CAD build for the part. Positions are in the model's coordinates, mm. Face numbers are marked on the shaded views. Round coordinates to 2 decimals unless told otherwise and drop trailing zeros. Order: outer loops, then holes, each group sorted by start corner. A loop starts at its lowest first (then second) coordinate and runs counter-clockwise, first axis right, second up. Notation, with made-up numbers: M -8.75,69.25 L 20.25,69.25 A28 cw 20.25,105.25 Z; hole C 44.25,31 d6. An arc over 180 degrees is marked long. Answer as a JSON object with one key per item and string values.
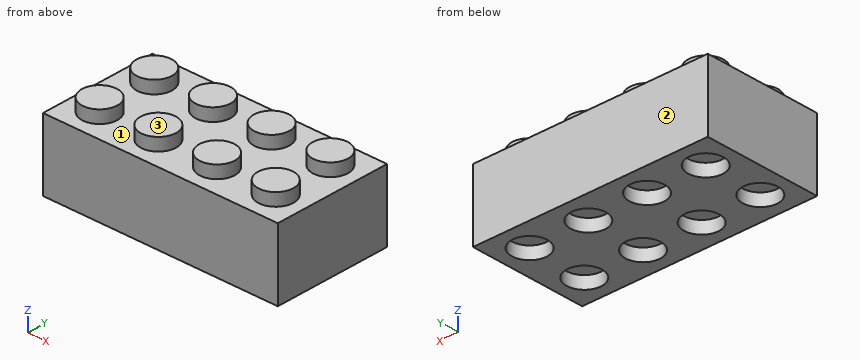
```python
from build123d import *

# Parameters (mm, degrees)
F1_DEPTH = 8
F3_W     = 8
F3_H     = 8
F3_R     = 2.4
F4_DEPTH = 1.7
F5_R     = 2.4
F6_DEPTH = 1.7


with BuildPart() as f1:
    # F0 (on Front) → F1 (new body)
    with BuildSketch(Plane.XZ):
        Polygon((-2.4, 9.6), (-4, 9.6), (-4, 0), (4, 0), (4, 9.6), (2.4, 9.6), (2.4, 11.3), (-2.4, 11.3), align=None)
    extrude(amount=F1_DEPTH)

    # F3 (on plane+point) → F4 (cut, through all)
    with BuildSketch(Plane.XY.offset(11.3)):
        with Locations((0, -4)):
            Rectangle(F3_W, F3_H)
        with Locations((0, -4)):
            Circle(F3_R, mode=Mode.SUBTRACT)
    extrude(amount=-F4_DEPTH, mode=Mode.SUBTRACT)

    # F5 (on Top) → F6 (cut)
    with BuildSketch(Plane.XY):
        with Locations((0, -4)):
            Circle(F5_R)
    extrude(amount=F6_DEPTH, mode=Mode.SUBTRACT)

    # F8: F1 across plane


with BuildPart() as f1_1:
    add(f1.part)
    add(f1.part.mirror(Plane.YZ.offset(4)))

    # F9: F1 across plane


with BuildPart() as f1_2:
    add(f1_1.part)
    add(f1_1.part.mirror(Plane.XZ))

    # F11: F1 across plane


with BuildPart() as f1_3:
    add(f1_2.part)
    add(f1_2.part.mirror(Plane.YZ.offset(12)))


solid = f1_3.part
```
Item 1: Saw through at A-A on x = 0. List the corners of the cut face in (y, z), and give its area (3 significant figures).
Worked answers:
{"outline": "M -8,0 L -6.4,0 L -6.4,1.7 L -1.6,1.7 L -1.6,0 L 1.6,0 L 1.6,1.7 L 6.4,1.7 L 6.4,0 L 8,0 L 8,9.6 L 6.4,9.6 L 6.4,11.3 L 1.6,11.3 L 1.6,9.6 L -1.6,9.6 L -1.6,11.3 L -6.4,11.3 L -6.4,9.6 L -8,9.6 Z", "area": "154 mm2"}
Item 2: Wall check: line 1 along X through (y, z) = (4, 0.5); line 2 along Y through (x, z) = (0, 0.75); line 3 along Z through (x, y) = (15, -2.5). Give the ranges that are in metal, low to high. Write a range as [from, to].
Worked answers:
{"line 1": "x = [-4, -2.4], [2.4, 5.6], [10.4, 13.6], [18.4, 21.6], [26.4, 28]", "line 2": "y = [-8, -6.4], [-1.6, 1.6], [6.4, 8]", "line 3": "z = [1.7, 11.3]"}
Item 3: Drop a flat-ended pin along its axis: pin 1 Ø1.4 at (x, y) = (15, -4.5) entering from -Z. Give the stop position or say it passes through.
Worked answers:
{"pin 1": "stops at z = 1.7"}
Item 4: Two-plate mould, pull along Y, no slides. Class the marked faces 1, 2 and 3: released by +Y, released by -Y, zero draft, split by the parting line, or undercut.
Worked answers:
{"face 1": "undercut", "face 2": "released by +Y", "face 3": "zero draft"}
Item 5: Saw through at B-B on y = 0. List the corners of the cut face in (x, z).
Worked answers:
{"outline": "M -4,0 L 28,0 L 28,9.6 L -4,9.6 Z"}
